from build123d import *

# Parameters (mm, degrees)
F0_W     = 19.05
F0_H     = 25.4
F1_DEPTH = 1.016
F2_SIZE  = 2.032
F3_SIZE  = 2.032
F4_R     = 0.762
F5_R     = 0.4573869554
F6_DEPTH = 17.78
F9_DEPTH = 0.889


# Not quite as in the source:
# - the program builds the solid bodies; features that only make, move or delete a surface that nothing else refers to are left out


with BuildPart() as f1:
    # F0 (on Top) → F1 (new body)
    with BuildSketch(Plane.XY):
        with Locations((9.525, 12.7)):
            Rectangle(F0_W, F0_H)
    extrude(amount=F1_DEPTH)

    # F2
    f2_edges = [f1.edges().sort_by_distance(p)[0] for p in [
        (0, 0, 0.508),
    ]]
    chamfer(f2_edges, length=F2_SIZE)

    # F3
    f3_edges = [f1.edges().sort_by_distance(p)[0] for p in [
        (19.05, 0, 0.508),
    ]]
    chamfer(f3_edges, length=F3_SIZE)

    # F4
    f4_edges = [f1.edges().sort_by_distance(p)[0] for p in [
        (19.05, 25.4, 0.508),
    ]]
    fillet(f4_edges, radius=F4_R)

    # F5 (on face) → F6 (join)
    with BuildSketch(Plane.XY.offset(1.016)):
        with Locations((3.5583837889, 23.701650244)):
            Circle(F5_R)
    extrude(amount=F6_DEPTH)

    # F8 (on face) → F9 (join)
    with BuildSketch(Plane.XY.offset(18.796)):
        with BuildLine():
            ThreePointArc((4.0157707443, 23.701650244), (3.9885840141, 23.5463099941), (3.9102557402, 23.4094363551))
            Line((3.9102557402, 23.4094363551), (15.3415361419, 23.4094363551))
            Line((15.3415361419, 23.4094363551), (15.3415361419, 24.0212995559))
            Line((15.3415361419, 24.0212995559), (3.8855338223, 24.0212995559))
            ThreePointArc((3.8855338223, 24.0212995559), (3.9819619899, 23.8742316295), (4.0157707443, 23.701650244))
        make_face()
        with BuildLine():
            Line((3.2065118376, 23.9938641329), (3.2065118376, 23.4094363551))
            Line((3.2065118376, 23.4094363551), (3.9102557402, 23.4094363551))
            ThreePointArc((3.9102557402, 23.4094363551), (3.9885840141, 23.5463099941), (4.0157707443, 23.701650244))
            ThreePointArc((4.0157707443, 23.701650244), (3.9819619899, 23.8742316295), (3.8855338223, 24.0212995559))
            Line((3.8855338223, 24.0212995559), (3.2312337555, 24.0212995559))
            ThreePointArc((3.2312337555, 24.0212995559), (3.2185957822, 24.0078314607), (3.2065118376, 23.9938641329))
        make_face()
    extrude(amount=F9_DEPTH)


solid = f1.part
Work out the finished part from the listing and answer in its coordinate system (mm). A direction names the side the tool comes from. Give positions to 0.01 mm unless a question says otherwise; leave off trailing zeros. Write each loop counter-clockwise with the first axis right and the second up, starting at its lowest first coordinate (ties: lowest second). Pieces come first, ordered by that corner, then holes. Notation, with made-up numbers: M 57.5,11.5 L 113.5,11.5 A29 ccw 113.5,42.5 Z; hole C 64.25,41 d9. An arc over 180 degrees is marked long. Answer as CSV lines item,"result".
Q1. A cutting plane is placed at A-A on x = 4.5. Write down the section's boundary in (y, z) (3 decimals), plus the area to 3 significant figures.
A:
outline,"M 0,0 L 25.4,0 L 25.4,1.016 L 0,1.016 Z; M 23.409,18.796 L 24.021,18.796 L 24.021,19.685 L 23.409,19.685 Z"
area,"26.4 mm²"
Q2. A tool of negligible diameter and unlimited length cuts with its end or side. For faces 1 (the flat face through (9, 23.409, 19)), 2 (the flat face through (9, 24.021, 19)), 3 (the flat face through (1.03, 1, 0.5)), from which of +Z, -Z, +X, -X, +Y, -Y can it reach the whole face along a straight path? Write none if from no direction.
A:
face 1,"+Z, +X, -X, -Y"
face 2,"+Z, +X, -X, +Y"
face 3,"+Z, -Z, -X, -Y"
Q3. Given P1, Ø1, axis at x = 9, z = 19, coming from the -Y side; P2, Ø2, axis at x = 15, y = 14, coming from the +Z side; P3, Ø1, axis at x = 9, z = 19, coming from the +Y side, each flat-ended and moving along its own axis, determine where each tip first touches the part or whether it passes through.
A:
P1,"stops at y = 23.41"
P2,"stops at z = 1.02"
P3,"stops at y = 24.02"
Q4. Find the intervals of material crossed by probe 1 along Z at (x, y) = (13, 4); probe 2 along Y at (x, z) = (6.25, 19.25); probe 3 along X at (y, z) = (23.5, 16.5), in increasing order. Write a range as [from, to].
A:
probe 1,"z = [0, 1.02]"
probe 2,"y = [23.41, 24.02]"
probe 3,"x = [3.15, 3.97]"
Q5. A cutting plane is placed at C-C on x = 16.25. Write down the section's boundary in (y, z).
A:
outline,"M 0,0 L 25.4,0 L 25.4,1.02 L 0,1.02 Z"
Q6. A cutting plane is placed at B-B on y = 19.25. Write down the section's boundary in (x, z), plus the area to 3 significant figures.
A:
outline,"M 0,0 L 19.05,0 L 19.05,1.02 L 0,1.02 Z"
area,"19.4 mm²"
Q7. A cutting plane is placed at D-D on z = 3.75. Write down the section's boundary in (x, y).
A:
outline,"C 3.56,23.7 d0.91"
